```python
from build123d import *

# Parameters (mm, degrees)
SKETCH1_W               = 77
SKETCH1_H               = 60
BOSS_EXTRUDE1_DEPTH     = 8
SKETCH3_W               = 60
SKETCH3_H               = 26
BOSS_EXTRUDE2_DEPTH     = 9
SKETCH4_R               = 4
CUT_EXTRUDE2_DEPTH      = 107.395488626
SKETCH5_W               = 34.3
SKETCH5_H               = 44
RECESS_DEPTH            = 1
ANGLES_IN_RECESS_DEPTH  = 44
SKETCH7_W               = 7
SKETCH7_H               = 60
WHERE_THE_BELT_GO_DEPTH = 1


with BuildPart() as part:
    # Sketch1 → Boss-Extrude1 (new body)
    with BuildSketch(Plane(origin=(0, 0, 0), x_dir=(1, 0, 0), z_dir=(0, 1, 0))):
        with Locations((38.5, 30)):
            Rectangle(SKETCH1_W, SKETCH1_H)
    extrude(amount=BOSS_EXTRUDE1_DEPTH)

    # Sketch3 → Boss-Extrude2 (add)
    with BuildSketch(Plane(origin=(77, 0, 0), x_dir=(0, 0, -1), z_dir=(1, 0, 0))):
        with Locations((30, -5)):
            Rectangle(SKETCH3_W, SKETCH3_H)
    extrude(amount=BOSS_EXTRUDE2_DEPTH)

    # Sketch4 → Cut-Extrude2 (cut, through all)
    with BuildSketch(Plane(origin=(86, 0, 0), x_dir=(0, 0, -1), z_dir=(1, 0, 0))):
        with Locations((8.5, -7)):
            Circle(SKETCH4_R)
        with Locations(Location((51.5, -7, 0), (0, 0, 180))):
            Circle(SKETCH4_R)
    extrude(amount=-CUT_EXTRUDE2_DEPTH, mode=Mode.SUBTRACT)

    # Sketch5 → recess (cut)
    with BuildSketch(Plane(origin=(0, 8, 0), x_dir=(1, 0, 0), z_dir=(0, 1, 0))):
        with Locations((43, 34)):
            Rectangle(SKETCH5_W, SKETCH5_H)
    extrude(amount=-RECESS_DEPTH, mode=Mode.SUBTRACT)

    # Sketch6 → Angles in recess (cut)
    with BuildSketch(Plane.XY.offset(-56)):
        Polygon((25.85, 7), (24.85, 8), (25.85, 8), align=None)
        Polygon((60.15, 8), (60.15, 7), (61.15, 8), align=None)
    extrude(amount=ANGLES_IN_RECESS_DEPTH, mode=Mode.SUBTRACT)

    # Sketch7 → where the belt go (cut)
    with BuildSketch(Plane.XZ):
        with Locations((38.5, -30)):
            Rectangle(SKETCH7_W, SKETCH7_H)
    extrude(amount=-WHERE_THE_BELT_GO_DEPTH, mode=Mode.SUBTRACT)


solid = part.part
```
Input: part model. Units: mm. Frame: model coordinates. A direction names the side the tool comes from. Coordinates: 2 decimals unless noted, no trailing zeros. Loops run counter-clockwise (first coordinate to the right, second up) from the corner with the lowest first, then second, coordinate; pieces in that order, holes last. Notation, with made-up numbers: (62.25, 14.25) -> (113.25, 14.25) arc R16 cw to (113.25, 37.25) -> close; hole circle Ø1 at (27.5, 17). An arc over 180 degrees is marked (long way). Use a Markdown table: item, result.
1) Pull-direction query (Z, two-part tool) for faces 1 (the flat face through (52, 1, -60)), 2 (the flat face through (59, 0, -30)), 3 (the flat face through (43, 7, -34)); classes: released by +Z, released by -Z, zero draft, split by the parting line, or undercut.
Results found:
| item | result |
|---|---|
| face 1 | released by -Z |
| face 2 | zero draft |
| face 3 | undercut |
2) Contact query for flat-ended pins moving along their axis: pin 1 (10.5 mm diameter, centred on y = -7, z = -51.5, fed in from -X); pin 2 (3 mm diameter, centred on y = 0.5, z = -8.5, fed in from -X); pin 3 (10.5 mm diameter, centred on x = 64.5, z = -43, fed in from -Y); pin 4 (10 mm diameter, centred on x = 51.5, z = -46.5, fed in from +Y). Output: stop coordinate, or through.
Results found:
| item | result |
|---|---|
| pin 1 | stops at x = 77 |
| pin 2 | stops at x = 0 |
| pin 3 | stops at y = 0 |
| pin 4 | stops at y = 7 |
3) Cut plane D-D (z = -39.5). Return the cut outline in (x, y).
Results found:
| item | result |
|---|---|
| outline | (0, 0) -> (35, 0) -> (35, 1) -> (42, 1) -> (42, 0) -> (77, 0) -> (77, -18) -> (86, -18) -> (86, 8) -> (61.15, 8) -> (60.15, 7) -> (25.85, 7) -> (24.85, 8) -> (0, 8) -> close |
4) Access query for faces 4 (the flat face through (77, -9, -30)), 5 (the flat face through (38, 1, -30)), 6 (the flat face through (42, 8, -10)). Directions: +Z, -Z, +X, -X, +Y, -Y. A direction counts if a zero-diameter tool reaches every point of the face in a straight line with its end or side. Return the directions, or none.
Results found:
| item | result |
|---|---|
| face 4 | +Z, -Z, -X, -Y |
| face 5 | +Z, -Z, -Y |
| face 6 | +Z, -Z, +X, -X, +Y |
5) Cut plane C-C (x = 48.5). Return the cut outline in (y, z).
Results found:
| item | result |
|---|---|
| outline | (0, -60) -> (8, -60) -> (8, -56) -> (7, -56) -> (7, -12) -> (8, -12) -> (8, 0) -> (0, 0) -> close |
6) Material intervals for line 1 along Y through (x, z) = (82.75, -8.5); line 2 along X through (y, z) = (0.5, -11); line 3 along Y through (x, z) = (53, -32), sorted ascending. Write a range as from..to.
Results found:
| item | result |
|---|---|
| line 1 | y = -18..-11, -3..8 |
| line 2 | x = 0..35, 42..86 |
| line 3 | y = 0..7 |
7) Cut plane B-B (y = -7). Return the cut outline in (x, z).
Results found:
| item | result |
|---|---|
| outline | (77, -60) -> (86, -60) -> (86, -55.5) -> (77, -55.5) -> close; (77, -47.5) -> (86, -47.5) -> (86, -12.5) -> (77, -12.5) -> close; (77, -4.5) -> (86, -4.5) -> (86, 0) -> (77, 0) -> close |
8) Cut plane A-A (z = -8.5). Return the cut outline in (x, y).
Results found:
| item | result |
|---|---|
| outline | (0, 0) -> (35, 0) -> (35, 1) -> (42, 1) -> (42, 0) -> (77, 0) -> (77, -3) -> (86, -3) -> (86, 8) -> (0, 8) -> close; (77, -18) -> (86, -18) -> (86, -11) -> (77, -11) -> close |
